Can you work these out from the model? Positions are in its coordinate system, mm. Round coordinates to 2 decimals unless told otherwise and drop trailing zeros. Loops run counter-clockwise (first coordinate to the right, second up) from the corner with the lowest first, then second, coordinate; pieces in that order, holes last. Notation, with made-up numbers: (-17, -39.75) -> (-3, -39.75) arc R24 ccw to (-3, -7.75) -> close; hole circle Ø7 at (62.25, -22.75). An arc over 180 degrees is marked (long way). Write item = value, one per line.
from build123d import *

# Parameters (mm, degrees)
SKETCH1_R               = 5
BOSS_EXTRUDE1_DEPTH     = 6
FILLET3_R               = 1
SKETCH2_R               = 2.5
CUT_EXTRUDE1_DEPTH      = 1
CUT_EXTRUDE1_DEPTH_BACK = 7
SKETCH3_R               = 1.25
CUT_EXTRUDE2_DEPTH      = 6.0000001
CUT_EXTRUDE2_DEPTH_BACK = 6


with BuildPart() as part:
    # Sketch1 → Boss-Extrude1 (new body)
    with BuildSketch(Plane.XY):
        Circle(SKETCH1_R)
    extrude(amount=BOSS_EXTRUDE1_DEPTH)

    # Fillet3
    fillet3_edges = [part.edges().sort_by_distance(p)[0] for p in [
        (-5, 0, 0),
        (-5, 0, 6),
    ]]
    fillet(fillet3_edges, radius=FILLET3_R)

    # Sketch2 → Cut-Extrude1 (cut, two sides)
    with BuildSketch(Plane.XY.offset(6)) as cut_extrude1_sk:
        Circle(SKETCH2_R)
    extrude(amount=CUT_EXTRUDE1_DEPTH, mode=Mode.SUBTRACT)
    extrude(cut_extrude1_sk.sketch, amount=-CUT_EXTRUDE1_DEPTH_BACK, mode=Mode.SUBTRACT)

    # Sketch3 → Cut-Extrude2 (cut, two sides)
    with BuildSketch(Plane(origin=(0, 0, 0), x_dir=(1, 0, 0), z_dir=(0, 1, 0))) as cut_extrude2_sk:
        with Locations((0, -3)):
            Circle(SKETCH3_R)
    extrude(amount=CUT_EXTRUDE2_DEPTH, mode=Mode.SUBTRACT)
    extrude(cut_extrude2_sk.sketch, amount=-CUT_EXTRUDE2_DEPTH_BACK, mode=Mode.SUBTRACT)


solid = part.part
1. Suppose I cut it at C-C, the plane z = 4. List the corners of the cut face in (x, y) for me, and give its area (3 significant figures).
Entries:
outline = (-0.75, -4.94) -> (-0.75, -2.38) arc R2.5 cw to (-0.75, 2.38) -> (-0.75, 4.94) arc R5 ccw to start; (0.75, -4.94) arc R5 ccw to (0.75, 4.94) -> (0.75, 2.38) arc R2.5 cw to (0.75, -2.38) -> close
area = 51.3 mm²
2. We'd pull the mould along Y, two halves only. Please class faces 1 (the cylindrical face through (-0.27, 3.57, 4.22)), 2 (the cylindrical face through (2.385, 0.751, 3.042)), 3 (the cylindrical face through (2.307, -4.436, 2.972)): released by +Y, released by -Y, zero draft, split by the parting line, or undercut.
Entries:
face_1 = zero draft
face_2 = undercut
face_3 = split by the parting line
3. I need wall thicknesses on line 1 (Z direction, x = 0, y = -2.8); line 2 (X direction, y = 3, z = 3); line 3 (Y direction, x = -2, z = 4.25). Which ranges of each line are inside material? Lowest first, please. Write a range as [from, to].
Entries:
line_1 = [0, 1.75], [4.25, 6]
line_2 = [-4, -1.25], [1.25, 4]
line_3 = [-4.58, -1.5], [1.5, 4.58]
4. Suppose I cut it at D-D, the plane z = 3. List the corners of the cut face in (x, y) for me, and give its area (3 significant figures).
Entries:
outline = (-1.25, -4.84) -> (-1.25, -2.17) arc R2.5 cw to (-1.25, 2.17) -> (-1.25, 4.84) arc R5 ccw to start; (1.25, -4.84) arc R5 ccw to (1.25, 4.84) -> (1.25, 2.17) arc R2.5 cw to (1.25, -2.17) -> close
area = 46.1 mm²
5. I'm going to push a flat-ended pin straight in: pin 1 (1.5 mm diameter, centred on x = -2.5, z = 4.5, fed in from +Y). Where does the tip first touch, or does it pass through?
Entries:
pin_1 = 4.68
6. Suppose I cut it at A-A, the plane x = 0. List the corners of the cut face in (y, z) for me, and give its area (3 significant figures).
Entries:
outline = (-5, 1) arc R1 ccw to (-4, 0) -> (-2.5, 0) -> (-2.5, 1.75) -> (-5, 1.75) -> close; (-5, 4.25) -> (-2.5, 4.25) -> (-2.5, 6) -> (-4, 6) arc R1 ccw to (-5, 5) -> close; (2.5, 0) -> (4, 0) arc R1 ccw to (5, 1) -> (5, 1.75) -> (2.5, 1.75) -> close; (2.5, 4.25) -> (5, 4.25) -> (5, 5) arc R1 ccw to (4, 6) -> (2.5, 6) -> close
area = 16.6 mm²
7. Suppose I cut it at B-B, the plane y = 0. List the corners of the cut face in (x, z) for me.
Entries:
outline = (-5, 1) arc R1 ccw to (-4, 0) -> (-2.5, 0) -> (-2.5, 6) -> (-4, 6) arc R1 ccw to (-5, 5) -> close; (2.5, 0) -> (4, 0) arc R1 ccw to (5, 1) -> (5, 5) arc R1 ccw to (4, 6) -> (2.5, 6) -> close
